Input: part model. Units: mm. Frame: model coordinates. Give positions to 0.01 mm unless a question says otherwise; leave off trailing zeros. Loops run counter-clockwise (first coordinate to the right, second up) from the corner with the lowest first, then second, coordinate; pieces in that order, holes last. Notation, with made-up numbers: (45, -7.75) - (73, -7.75) arc R17 ccw to (73, 23.25) - close; hole circle Ø8 at (47.25, 79). An arc over 180 degrees is marked (long way). Answer as a JSON object with one key per item and string values.
from build123d import *

# Parameters (mm, degrees)
SKETCH_1_W                                 = 307
SKETCH_1_H                                 = 200
EXTRUDE_1_DEPTH                            = 3
SKETCH_2_W                                 = 84
SKETCH_2_H                                 = 33
CUT_EXTRUDE_1_DEPTH                        = 3
PATTERN_LINEAR_1_COUNT                     = 2
PATTERN_LINEAR_1_PITCH                     = 170
PATTERN_LINEAR_1_COUNT_DIR2                = 2
PATTERN_LINEAR_1_PITCH_DIR2                = 167
SKETCH_6_R                                 = 12.5
CUT_EXTRUDE_2_DEPTH                        = 3
FILLET_1_R                                 = 10
SKETCH_11_R                                = 1.5
CUT_EXTRUDE_3_DEPTH                        = 10
SKETCH_11_3_R                              = 1.5
CUT_EXTRUDE_4_DEPTH                        = 10
MIRROR_2_AT_THE_SECOND_PLANE_COPY_1_SKET_R = 1.5
MIRROR_2_AT_THE_SECOND_PLANE_COPY_1_DEPTH  = 10
MIRROR_2_AT_THE_SECOND_PLANE_COPY_2_SKET_R = 1.5
MIRROR_2_AT_THE_SECOND_PLANE_COPY_2_DEPTH  = 10


with BuildPart() as part:
    # Sketch 1 → Extrude 1 (new body)
    with BuildSketch(Plane(origin=(0, 0, 0), x_dir=(1, 0, 0), z_dir=(0, 1, 0))):
        with Locations((-43.995626822, 46.034985423)):
            Rectangle(SKETCH_1_W, SKETCH_1_H)
    extrude(amount=EXTRUDE_1_DEPTH)

    # Sketch 2 → Cut-Extrude 1 (cut)
    with BuildSketch(Plane(origin=(0, 3, 0), x_dir=(1, 0, 0), z_dir=(0, 1, 0))):
        with Locations((-128.495626822, 129.534985423)):
            Rectangle(SKETCH_2_W, SKETCH_2_H)
    cut_extrude_1 = extrude(amount=-CUT_EXTRUDE_1_DEPTH, mode=Mode.SUBTRACT)

    # Pattern Linear 1: Cut-Extrude 1 2 × 2
    with Locations(*[(i * PATTERN_LINEAR_1_PITCH, 0, j * PATTERN_LINEAR_1_PITCH_DIR2) for i in range(PATTERN_LINEAR_1_COUNT) for j in range(PATTERN_LINEAR_1_COUNT_DIR2) if (i, j) != (0, 0)]):
        add(cut_extrude_1, mode=Mode.SUBTRACT)

    # Sketch 6 → Cut-Extrude 2 (cut)
    with BuildSketch(Plane(origin=(0, 3, 0), x_dir=(1, 0, 0), z_dir=(0, 1, 0))):
        with Locations(Location((-43.995626822, 46.034985423, 0), (0, 0, 270))):
            Circle(SKETCH_6_R)
    extrude(amount=-CUT_EXTRUDE_2_DEPTH, mode=Mode.SUBTRACT)

    # Fillet 1
    fillet_1_edges = [part.edges().sort_by_distance(p)[0] for p in [
        (109.504373178, 1.5, 53.965014577),
        (-197.495626822, 1.5, 53.965014577),
        (-197.495626822, 1.5, -146.034985423),
        (109.504373178, 1.5, -146.034985423),
    ]]
    fillet(fillet_1_edges, radius=FILLET_1_R)

    # Sketch 11 → Cut-Extrude 3 (cut)
    with BuildSketch(Plane.XZ):
        with Locations(Location((26.504373178, 14.465014577, 0), (0, 0, 270))):
            Circle(SKETCH_11_R)
        with Locations(Location((56.504373178, 14.465014577, 0), (0, 0, 270))):
            Circle(SKETCH_11_R)
    cut_extrude_3 = extrude(amount=-CUT_EXTRUDE_3_DEPTH, mode=Mode.SUBTRACT)

    # Sketch 11_3 → Cut-Extrude 4 (cut)
    with BuildSketch(Plane.XZ):
        with Locations(Location((26.504373178, 14.465014577, 0), (0, 0, 270))):
            Circle(SKETCH_11_3_R)
        with Locations(Location((56.504373178, 14.465014577, 0), (0, 0, 270))):
            Circle(SKETCH_11_3_R)
        with Locations(Location((56.504373178, -0.534985423, 0), (0, 0, 270))):
            Circle(SKETCH_11_3_R)
        with Locations(Location((26.504373178, -0.534985423, 0), (0, 0, 270))):
            Circle(SKETCH_11_3_R)
    cut_extrude_4 = extrude(amount=-CUT_EXTRUDE_4_DEPTH, mode=Mode.SUBTRACT)

    # Mirror 2: Cut-Extrude 3, Cut-Extrude 4 across plane
    add(cut_extrude_3.mirror(Plane(origin=(-43.995626822, 0, 0), x_dir=(0, 0, 1), z_dir=(1, 0, 0))), mode=Mode.SUBTRACT)
    add(cut_extrude_4.mirror(Plane(origin=(-43.995626822, 0, 0), x_dir=(0, 0, 1), z_dir=(1, 0, 0))), mode=Mode.SUBTRACT)

    # Mirror 2 at the second plane: Cut-Extrude 3, Cut-Extrude 4 across plane
    add(cut_extrude_3.mirror(Plane(origin=(0, 0, -46.034985423), x_dir=(1, 0, 0), z_dir=(0, 0, -1))), mode=Mode.SUBTRACT)
    add(cut_extrude_4.mirror(Plane(origin=(0, 0, -46.034985423), x_dir=(1, 0, 0), z_dir=(0, 0, -1))), mode=Mode.SUBTRACT)

    # Mirror 2 at the second plane copy 1 sket → Mirror 2 at the second plane copy 1 (cut)
    with BuildSketch(Plane(origin=(-87.991253644, 0, -92.069970845), x_dir=(-1, 0, 0), z_dir=(0, -1, 0))):
        with Locations(Location((26.504373178, 14.465014577, 0), (0, 0, 270))):
            Circle(MIRROR_2_AT_THE_SECOND_PLANE_COPY_1_SKET_R)
        with Locations(Location((56.504373178, 14.465014577, 0), (0, 0, 270))):
            Circle(MIRROR_2_AT_THE_SECOND_PLANE_COPY_1_SKET_R)
    extrude(amount=-MIRROR_2_AT_THE_SECOND_PLANE_COPY_1_DEPTH, mode=Mode.SUBTRACT)

    # Mirror 2 at the second plane copy 2 sket → Mirror 2 at the second plane copy 2 (cut)
    with BuildSketch(Plane(origin=(-87.991253644, 0, -92.069970845), x_dir=(-1, 0, 0), z_dir=(0, -1, 0))):
        with Locations(Location((26.504373178, 14.465014577, 0), (0, 0, 270))):
            Circle(MIRROR_2_AT_THE_SECOND_PLANE_COPY_2_SKET_R)
        with Locations(Location((56.504373178, 14.465014577, 0), (0, 0, 270))):
            Circle(MIRROR_2_AT_THE_SECOND_PLANE_COPY_2_SKET_R)
        with Locations(Location((56.504373178, -0.534985423, 0), (0, 0, 270))):
            Circle(MIRROR_2_AT_THE_SECOND_PLANE_COPY_2_SKET_R)
        with Locations(Location((26.504373178, -0.534985423, 0), (0, 0, 270))):
            Circle(MIRROR_2_AT_THE_SECOND_PLANE_COPY_2_SKET_R)
    extrude(amount=-MIRROR_2_AT_THE_SECOND_PLANE_COPY_2_DEPTH, mode=Mode.SUBTRACT)


solid = part.part
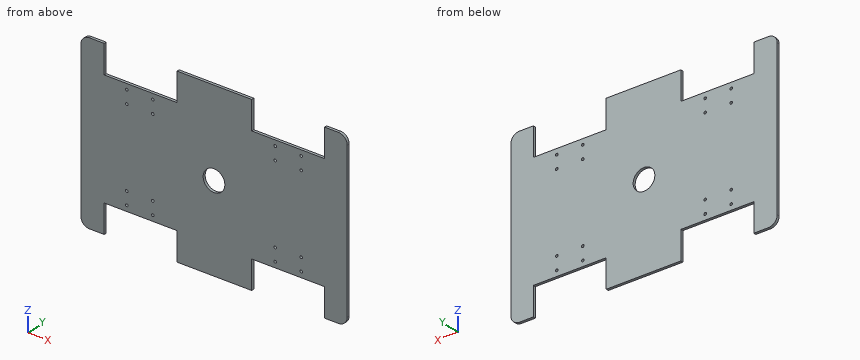
Item 1: Material intervals for line 1 (X direction, y = 2.2, z = -127.5); line 2 (Z direction, x = -45, y = 2.55); line 3 (Z direction, x = -125, y = 1.05), sorted ascending. Write a range as [from, to].
Geometry check:
{"line 1": "x = [-197.5, -170.5], [-86.5, -0.5], [83.5, 109.5]", "line 2": "z = [-146.03, -58.49], [-33.58, 53.97]", "line 3": "z = [-113.03, 20.97]"}
Item 2: Cut plane C-C (z = -39). Return loops of the section in (x, y), then the cut area to 3 significant figures.
Geometry check:
{"outline": "(-197.5, 0) - (-54.33, 0) - (-54.33, 3) - (-197.5, 3) - close; (-33.66, 0) - (109.5, 0) - (109.5, 3) - (-33.66, 3) - close", "area": "859 mm2"}
Item 3: Cut plane B-B (x = -47). Return loops of the section in (y, z).
Geometry check:
{"outline": "(0, -146.03) - (3, -146.03) - (3, -58.17) - (0, -58.17) - close; (0, -33.9) - (3, -33.9) - (3, 53.97) - (0, 53.97) - close"}
Item 4: Cut plane D-D (x = 64). Return loops of the section in (y, z).
Geometry check:
{"outline": "(0, -113.03) - (3, -113.03) - (3, 20.97) - (0, 20.97) - close"}
Item 5: Contact query for a flat-ended pin moving along its axis: P1, Ø0.9, axis at x = 58.5, y = 1, coming from the +Z side (3 decimals). Output: stop coordinate, or through.
Geometry check:
{"P1": "stops at z = 20.965"}
Item 6: Cut plane A-A (z = -119). Return loops of the section in (x, y), then the cut area to 3 significant figures.
Geometry check:
{"outline": "(-197.5, 0) - (-170.5, 0) - (-170.5, 3) - (-197.5, 3) - close; (-86.5, 0) - (-0.5, 0) - (-0.5, 3) - (-86.5, 3) - close; (83.5, 0) - (109.5, 0) - (109.5, 3) - (83.5, 3) - close", "area": "417 mm2"}
